Could you check a few things on this model? Use its own coordinates, in mm. Give positions to 0.01 mm unless a question says otherwise; leave off trailing zeros. Loops run counter-clockwise (first coordinate to the right, second up) from the corner with the lowest first, then second, coordinate; pieces in that order, holes last. Notation, with made-up numbers: (-34.75, 34.5) -> (-0.75, 34.5) arc R29 cw to (-0.75, 63.5) -> close; hole circle Ø3 at (-14, -28.5). An arc over 180 degrees is marked (long way). Put each result on its own line as item: value.
```python
from build123d import *

# Parameters (mm, degrees)
SKETCH_1_W                     = 73
SKETCH_1_H                     = 53
EXTRUDE_1_DEPTH                = 1.5
FILLET_1_R                     = 2
SKETCH_2_R                     = 1.6
CUT_EXTRUDE_1_DEPTH            = 46.130366717
PATTERN_LINEAR_1_COUNT         = 2
PATTERN_LINEAR_1_PITCH         = 60
PATTERN_LINEAR_1_COUNT_DIR2    = 2
PATTERN_LINEAR_1_PITCH_DIR2    = 40
SKETCH_3_W                     = 8
SKETCH_3_H                     = 12
CUT_EXTRUDE_2_DEPTH            = 46.130366717
FILLET_2_R                     = 1
PATTERN_LINEAR_2_COUNT         = 2
PATTERN_LINEAR_2_PITCH         = 20
FILLET_2_OF_PATTERN_LINEAR_2_R = 1


with BuildPart() as part:
    # 草图1 → 凸台-拉伸1 (new body)
    with BuildSketch(Plane(origin=(0, 0, 0), x_dir=(1, 0, 0), z_dir=(0, 1, 0))):
        Rectangle(SKETCH_1_W, SKETCH_1_H)
    extrude(amount=EXTRUDE_1_DEPTH)

    # 圆角1
    fillet_1_edges = [part.edges().sort_by_distance(p)[0] for p in [
        (-36.5, 0.75, -26.5),
        (36.5, 0.75, -26.5),
        (36.5, 0.75, 26.5),
        (-36.5, 0.75, 26.5),
    ]]
    fillet(fillet_1_edges, radius=FILLET_1_R)

    # 草图2 → 切除-拉伸1 (cut, through all)
    with BuildSketch(Plane(origin=(0, 1.5, 0), x_dir=(1, 0, 0), z_dir=(0, 1, 0))):
        with Locations(Location((-30, 20, 0), (0, 0, 270))):
            Circle(SKETCH_2_R)
    cut_extrude_1 = extrude(amount=-CUT_EXTRUDE_1_DEPTH, mode=Mode.SUBTRACT)

    # 阵列(线性)1: Cut-Extrude 1 2 × 2
    with Locations(*[(i * PATTERN_LINEAR_1_PITCH, 0, j * PATTERN_LINEAR_1_PITCH_DIR2) for i in range(PATTERN_LINEAR_1_COUNT) for j in range(PATTERN_LINEAR_1_COUNT_DIR2) if (i, j) != (0, 0)]):
        add(cut_extrude_1, mode=Mode.SUBTRACT)

    # 草图3 → 切除-拉伸2 (cut, through all)
    with BuildSketch(Plane(origin=(0, 1.5, 0), x_dir=(1, 0, 0), z_dir=(0, 1, 0))):
        with Locations((27.5, 10)):
            Rectangle(SKETCH_3_W, SKETCH_3_H)
    cut_extrude_2 = extrude(amount=-CUT_EXTRUDE_2_DEPTH, mode=Mode.SUBTRACT)

    # 圆角2
    fillet_2_edges = [part.edges().sort_by_distance(p)[0] for p in [
        (23.5, 0.75, -4),
        (23.5, 0.75, -16),
        (31.5, 0.75, -16),
        (31.5, 0.75, -4),
    ]]
    fillet(fillet_2_edges, radius=FILLET_2_R)

    # 阵列(线性)2: 切除-拉伸2 ×2
    with Locations(*[(0, 0, i * PATTERN_LINEAR_2_PITCH) for i in range(1, PATTERN_LINEAR_2_COUNT)]):
        add(cut_extrude_2, mode=Mode.SUBTRACT)

    # 圆角2 of 阵列(线性)2
    fillet_2_of_pattern_linear_2_edges = [part.edges().sort_by_distance(p)[0] for p in [
        (23.5, 0.75, 16),
        (23.5, 0.75, 4),
        (31.5, 0.75, 4),
        (31.5, 0.75, 16),
    ]]
    fillet(fillet_2_of_pattern_linear_2_edges, radius=FILLET_2_OF_PATTERN_LINEAR_2_R)


solid = part.part
```
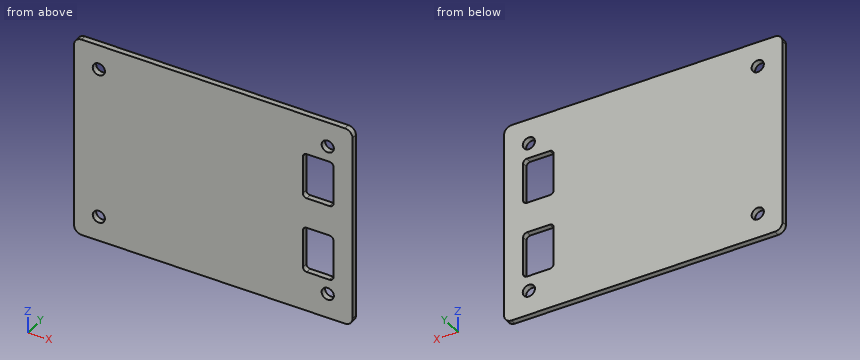
1. If we section it at D-D (z = -8): List the corners of the cut face in (x, y) for me, then the cut area to 3 significant figures.
Recorded:
outline: (-36.5, 0) -> (23.5, 0) -> (23.5, 1.5) -> (-36.5, 1.5) -> close; (31.5, 0) -> (36.5, 0) -> (36.5, 1.5) -> (31.5, 1.5) -> close
area: 97.5 mm^2
2. If we section it at A-A (z = -20): List the corners of the cut face in (x, y) for me, then the cut area to 3 significant figures.
Recorded:
outline: (-36.5, 0) -> (-31.6, 0) -> (-31.6, 1.5) -> (-36.5, 1.5) -> close; (-28.4, 0) -> (28.4, 0) -> (28.4, 1.5) -> (-28.4, 1.5) -> close; (31.6, 0) -> (36.5, 0) -> (36.5, 1.5) -> (31.6, 1.5) -> close
area: 99.9 mm^2
3. I need wall thicknesses on line 1 (Z direction, x = 26, y = 1.45); line 2 (X direction, y = 0.95, z = 20); line 3 (X direction, y = 1.1, z = -11). Which ranges of each line are inside material? Lowest first, please.
Recorded:
line 1: z = -26.5 to -16, -4 to 4, 16 to 26.5
line 2: x = -36.5 to -31.6, -28.4 to 28.4, 31.6 to 36.5
line 3: x = -36.5 to 23.5, 31.5 to 36.5
4. If we section it at B-B (y = 0.3): List the corners of the cut face in (x, z) for me.
Recorded:
outline: (-36.5, -24.5) arc R2 ccw to (-34.5, -26.5) -> (34.5, -26.5) arc R2 ccw to (36.5, -24.5) -> (36.5, 24.5) arc R2 ccw to (34.5, 26.5) -> (-34.5, 26.5) arc R2 ccw to (-36.5, 24.5) -> close; hole circle Ø3.2 at (-30, -20); hole circle Ø3.2 at (-30, 20); hole (23.5, -15) arc R1 ccw to (24.5, -16) -> (30.5, -16) arc R1 ccw to (31.5, -15) -> (31.5, -5) arc R1 ccw to (30.5, -4) -> (24.5, -4) arc R1 ccw to (23.5, -5) -> close; hole (23.5, 5) arc R1 ccw to (24.5, 4) -> (30.5, 4) arc R1 ccw to (31.5, 5) -> (31.5, 15) arc R1 ccw to (30.5, 16) -> (24.5, 16) arc R1 ccw to (23.5, 15) -> close; hole circle Ø3.2 at (30, -20); hole circle Ø3.2 at (30, 20)
5. If we section it at C-C (x = -30): List the corners of the cut face in (y, z) for me, then the cut area to 3 significant figures.
Recorded:
outline: (0, -26.5) -> (1.5, -26.5) -> (1.5, -21.6) -> (0, -21.6) -> close; (0, -18.4) -> (1.5, -18.4) -> (1.5, 18.4) -> (0, 18.4) -> close; (0, 21.6) -> (1.5, 21.6) -> (1.5, 26.5) -> (0, 26.5) -> close
area: 69.9 mm^2
